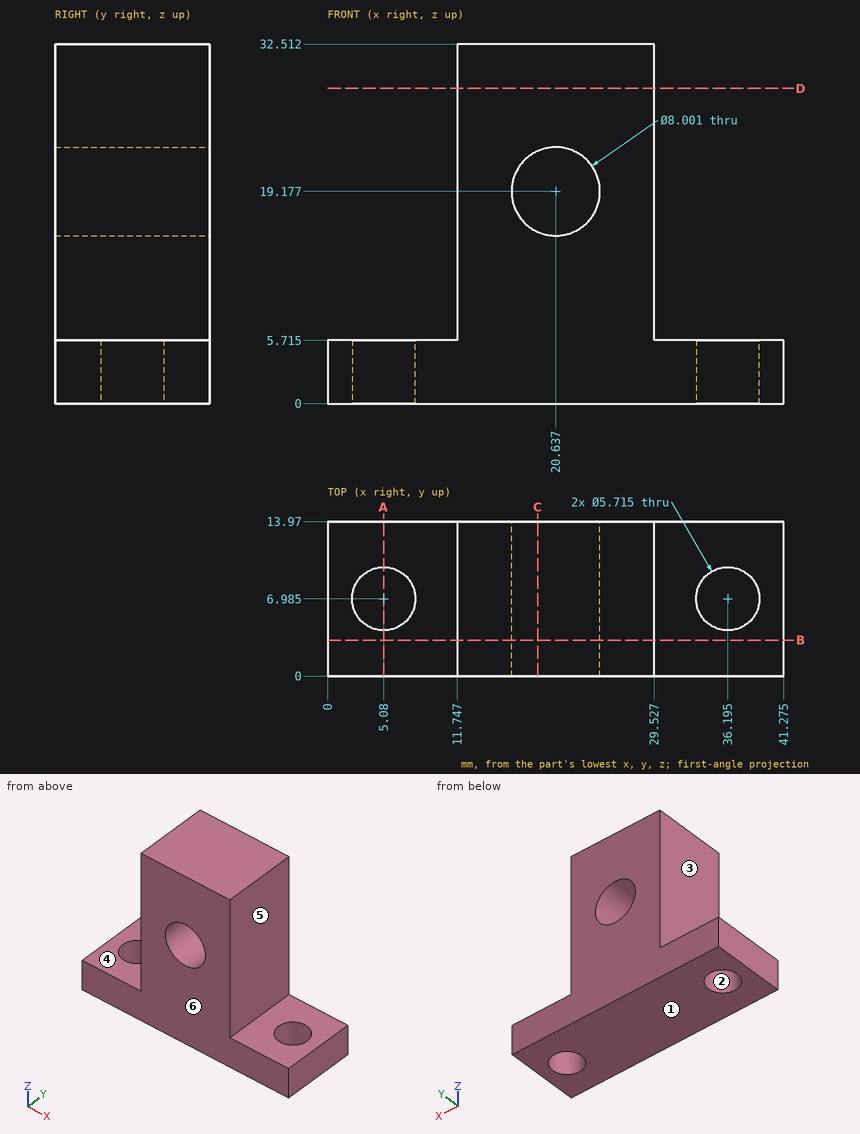
The drawing under review shows one solid part. Ordinate dimensions are in mm from its lowest x, y, z. A direction names the side the tool comes from. Give positions to 0.01 mm unless a question says otherwise; leave off trailing zeros. Write each loop counter-clockwise with the first axis right and the second up, starting at its lowest first coordinate (ties: lowest second). Pieces come first, ordered by that corner, then holes. Notation, with made-up numbers: (77.5, -38) - (107.5, -38) arc R19 ccw to (107.5, -19) - close; hole circle Ø10 at (-21, 56). An arc over 180 degrees is marked (long way). Answer in a Markdown table with one row per item. Add a question column.
1. Draft analysis for pull direction X (two halves, no side actions). For the marked faces 1, 2 and 3, state which applies: +X half, -X half, draft (parallel to the pull), parting line (faces both ways), or undercut.
2. We need section D-D on z = 28.5. Write out the cut boundary in (x, y).
3. Wall thickness on line 1 along X through (y, z) = (10.25, 19) (1 decimal); line 2 along Y through (x, z) = (5, 1); line 3 along X through (y, z) = (12.75, 7.5): over which ranges is each line inside the solid? List them lowest first. Write a range as [from, to].
4. Insertion check: P1, Ø1, axis at y = 8, z = 23.5, coming from the -X side; P2, Ø5, axis at x = 5.08, y = 6.985, coming from the +Z side; P3, Ø1.5, axis at y = 8.5, z = 22, coming from the +X side; P4, Ø6, axis at x = 3, y = 7.5, coming from the +Z side (1 decimal). Each pin has a flat end and moves straight along its axis. Give the tip position at first contact, or say it passes through.
5. We need section A-A on x = 5.08. Write out the cut boundary in (y, z) (1 decimal).
6. We need section B-B on y = 3.25. Write out the cut boundary in (x, z) (1 decimal), then the cut area to 3 significant figures.
7. We need section C-C on x = 19. Write out the cut boundary in (y, z).
8. Tool access review of the marked faces 4, 5 and 6: name each direction out of +Z, -Z, +X, -X, +Y, -Y from which nothing blocks a thin tool from reaching the whole face with its end or side.
Ans:
| question | item | result |
|---|---|---|
| 1 | face 1 | draft |
| 1 | face 2 | undercut |
| 1 | face 3 | -X half |
| 2 | outline | (11.75, 0) - (29.53, 0) - (29.53, 13.97) - (11.75, 13.97) - close |
| 3 | line 1 | x = [11.7, 16.6], [24.6, 29.5] |
| 3 | line 2 | y = [0, 4.13], [9.84, 13.97] |
| 3 | line 3 | x = [11.75, 29.53] |
| 4 | P1 | stops at x = 11.75 |
| 4 | P2 | passes through |
| 4 | P3 | stops at x = 29.53 |
| 4 | P4 | stops at z = 5.7 |
| 5 | outline | (0, 0) - (4.1, 0) - (4.1, 5.7) - (0, 5.7) - close; (9.8, 0) - (14, 0) - (14, 5.7) - (9.8, 5.7) - close |
| 6 | outline | (0, 0) - (41.3, 0) - (41.3, 5.7) - (29.5, 5.7) - (29.5, 32.5) - (11.7, 32.5) - (11.7, 5.7) - (0, 5.7) - close; hole circle Ø8 at (20.6, 19.2) |
| 6 | area | 662 mm^2 |
| 7 | outline | (0, 0) - (13.97, 0) - (13.97, 15.53) - (0, 15.53) - close; (0, 22.83) - (13.97, 22.83) - (13.97, 32.51) - (0, 32.51) - close |
| 8 | face 4 | +Z, -X, +Y, -Y |
| 8 | face 5 | +Z, +X, +Y, -Y |
| 8 | face 6 | +Z, -Z, +X, -X, -Y |
